Source: CAD feature listing. Evaluate the final solid. Frame: model axes, mm. Face numbers are marked on the shaded views. A direction names the side the tool comes from. Give positions to 0.01 mm unless a question says otherwise; leave off trailing zeros. Order: outer loops, then holes, each group sorted by start corner. A loop starts at its lowest first (then second) coordinate and runs counter-clockwise, first axis right, second up.
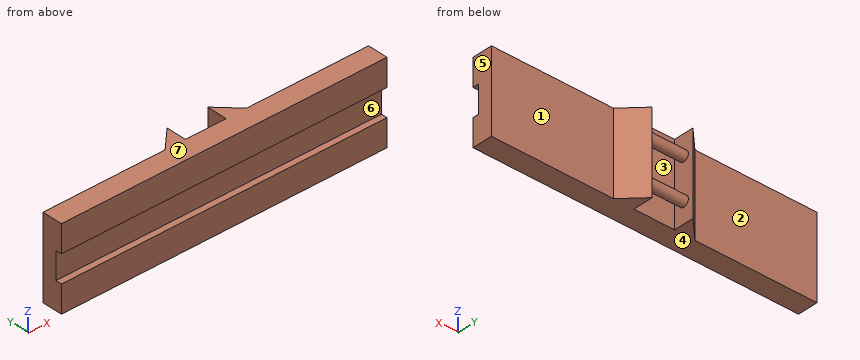
Autodesk Inventor part; units mm, degrees
ref_plane "YZ Plane" through (0, 0, 0) normal (1, 0, 0) x (0, 1, 0)
ref_plane "XZ Plane" through (0, 0, 0) normal (0, 1, 0) x (-1, 0, 0)
ref_plane "XY Plane" through (0, 0, 0) normal (0, 0, 1) x (1, 0, 0)
sketch "Sketch1" plane through (0, 0, 0) normal (0, 0, 1) x (1, 0, 0)
  line L0 (-1, 2) -> (-2, 1)
  line L1 (1, 2) -> (2, 1)
  line L2 (-1, 2) -> (-1, 1)
  line L3 (-1, 1) -> (1, 1)
  line L4 (1, 1) -> (1, 2)
  line L5 (0, 0) -> (8, 0)
  line L6 (8, 0) -> (8, 1)
  line L7 (8, 1) -> (2, 1)
  line L8 (0, 0) -> (-8, 0)
  line L9 (-8, 0) -> (-8, 1)
  line L10 (-8, 1) -> (-2, 1)
  dimension "d7" = 2
  dimension "d8" = 1
  dimension "d9" = 2
  dimension "d29" = 8
  dimension "d30" = 8
extrude "Extrusion1" add sketch "Sketch1" along normal blind 4
sketch "Sketch2" plane through (-1, 1, 0) normal (1, 0, 0) x (0, 0, -1)
  line L0 (0, 0) -> (0, 1)
  line L1 (-4, 0) -> (-4, 1)
  circle A0 centre (-1, 0.5) radius 0.25
  circle A1 centre (-3, 0.5) radius 0.25
  point P0 (0, -1)
  dimension "d14" = 0.5
  dimension "d15" = 0.5
extrude "Extrusion2" add sketch "Sketch2" along normal blind 2 contours A0
sketch "Sketch3" plane through (-1, 1, 0) normal (1, 0, 0) x (0, 0, -1)
  line L0 (-4, 0) -> (-4, 1)
  circle A0 centre (-3, 0.5) radius 0.25
  point P0 (0, -1)
  dimension "d19" = 0.5
extrude "Extrusion3" add sketch "Sketch3" along normal blind 2
sketch "Sketch4" plane through (7, 0, 0) normal (1, 0, 0) x (0, 0, -1)
  line L0 (0, 0) -> (-1.3333, 0)
  line L1 (-1.3333, 0) -> (-1.3333, 0.3)
  line L2 (-1.3333, 0.3) -> (-2.6667, 0.3)
  line L3 (-2.6667, 0.3) -> (-2.6667, 0)
  point P0 (-4, 0)
  dimension "d22" = 1.3333
  dimension "d23" = 1.3333
  dimension "d24" = 0.3
split "Split1" [suppressed]
sketch "Sketch5" plane through (-1, 1, 0) normal (1, 0, 0) x (0, 0, -1)
  line L0 (0, 0) -> (0, 1)
  circle A0 centre (-1, 0.5) radius 0.25
  circle A1 centre (-3, 0.5) radius 0.25
  point P0 (0, -1)
  dimension "d25" = 1
  dimension "d26" = 2
sketch "Sketch6" plane through (-1, 1, 0) normal (1, 0, 0) x (0, 0, -1)
  line L0 (0, 1) -> (-4, 1)
  circle A0 centre (-1, 0.5) radius 0.25
  point P0 (0, -1)
  dimension "d27" = 0.5
sketch "Sketch8" plane through (0, 0, 4) normal (0, 0, 1) x (1, 0, 0)
  point P0 (0, 0)
sketch "Sketch9" plane through (0, 0, 4) normal (0, 0, 1) x (1, 0, 0)
  point P0 (0, 0)
sketch "Sketch10" plane through (0, 0, 0) normal (0, 0, -1) x (-1, 0, 0)
  point P0 (0, 0)
sketch "Sketch11" plane through (-8, 0, 0) normal (-1, 0, 0) x (0, 0, 1)
  line L0 (2.6667, 0) -> (2.6667, 0.3)
  line L1 (2.6667, 0.3) -> (1.3333, 0.3)
  line L2 (1.3333, 0.3) -> (1.3333, 0)
  line L3 (2.6667, 0) -> (4, 0)
  point P0 (0, 0)
  dimension "d31" = 1.3333
  dimension "d32" = 1.3333
  dimension "d33" = 0.3
split body "Split2" sketch "Sketch11" result one side removed curves L3 L0 L1 L2 removed pieces at (-2.6667, 0.1, 1.7778)
properties part number "Tank Tread link A"
(1) Pin query (flat end, axial travel): pin 1 Ø1.5 at (x, z) = (-2.5, 1) entering from +Y; pin 2 Ø0.5 at (y, z) = (1.5, 2.5) entering from -X; pin 3 Ø2 at (x, z) = (-6.5, 2) entering from +Y; pin 4 Ø1.5 at (x, z) = (0.5, 3) entering from -Y. Return the tip coordinate at first contact, or that it passes through.
(2) Section B-B, the plane x = 4.5. Return loops of the section in (y, z), plus the area to 3 significant figures.
(3) Section A-A, the plane z = 1. Return loops of the section in (x, y), plus the area to 3 significant figures.
(4) Draft query along Z for the marked faces 5, 6 and 7. Return one class per face: +Z half, -Z half, draft (parallel to the pull), parting line (faces both ways), or undercut.
(5) Access query for the marked faces 1, 2, 3 and 4. Directions: +Z, -Z, +X, -X, +Y, -Y. A direction counts if a zero-diameter tool reaches every point of the face in a straight line with its end or side. Return the directions, or none.
(6) Line query: line 1 along Z through (x, y) = (2.25, 0.1); line 2 along Y through (x, z) = (-3.75, 1.5); line 3 along Y through (x, z) = (-6.5, 3.7). Output: solid intervals per line, ascending.
(7) Section C-C, the plane y = 1.5. Return loops of the section in (x, z).
Checks:
1. pin 1: stops at y = 1.25
1. pin 2: stops at x = -1.75
1. pin 3: stops at y = 1
1. pin 4: stops at y = 0
2. outline: (0, 0) - (1, 0) - (1, 4) - (0, 4) - (0, 2.67) - (0.3, 2.67) - (0.3, 1.33) - (0, 1.33) - close
2. area: 3.60 mm2
3. outline: (-8, 0) - (8, 0) - (8, 1) - (2, 1) - (1, 2) - (1, 1.75) - (-1, 1.75) - (-1, 2) - (-2, 1) - (-8, 1) - close; hole (-1, 1) - (1, 1) - (1, 1.25) - (-1, 1.25) - close
3. area: 18.0 mm2
4. face 5: draft
4. face 6: undercut
4. face 7: +Z half
5. face 1: +Z, -Z, +X, +Y
5. face 2: +Z, -Z, -X, +Y
5. face 3: +Z, -Z
5. face 4: -Z, +X, -X, +Y, -Y
6. line 1: z = 0 to 1.33, 2.67 to 4
6. line 2: y = 0.3 to 1
6. line 3: y = 0 to 1
7. outline: (-1.5, 0) - (-1, 0) - (-1, 0.75) - (1, 0.75) - (1, 0) - (1.5, 0) - (1.5, 4) - (1, 4) - (1, 3.25) - (-1, 3.25) - (-1, 4) - (-1.5, 4) - close; hole (-1, 1.25) - (1, 1.25) - (1, 2.75) - (-1, 2.75) - close
